Verification items for the finished model (mm, model axes). Face numbers are marked on the shaded views. A direction names the side the tool comes from. Coordinates: 2 decimals unless noted, no trailing zeros. Order: outer loops, then holes, each group sorted by start corner. A loop starts at its lowest first (then second) coordinate and runs counter-clockwise, first axis right, second up. Notation, with made-up numbers: M 54.25,49.25 L 73.25,49.25 A31 ccw 73.25,88.25 Z; hole C -29.5,-1.75 d4. An arc over 180 degrees is marked long. Return JSON: item names as keys, results as strings. Group by question number.
Q1. Access from +Z, -Z, +X, -X, +Y, -Y to the whole of each face (thin tool, end or side, straight path). Record for the marked faces 5, 6 and 7.
Q2. Section check C-C, the plane z = 2.25. Enter the section's corners in (x, y) (3 decimals).
Q3. Section check A-A, the plane y = -11. Enter the section's corners in (x, z), then the cut area to 3 significant figures.
Q4. Section check D-D, the plane x = 16. Enter the section's corners in (y, z) (3 decimals).
Q5. Thickness scan on probe 1 along Y at (x, z) = (-8, 15.25) (3 decimals); probe 2 along Y at (x, z) = (-12.5, 3.5) (3 decimals); probe 3 along Z at (x, y) = (8.5, 11). Record the ranges inside material, lowest first.
Q6. Mould release check, pull along X, two halves, no side actions. Record for the marked faces 1, 2, 3 and 4: pulls with the +X half, pulls with the -X half, needs draft (parallel to the pull), parting line crosses it, or undercut.
Q7. Go/stop test with flat-tipped pins: pin 1 Ø20 at (x, y) = (-9, -1.5) entering from +Z; pin 2 Ø8 at (y, z) = (-21.5, 9.5) entering from -X; pin 3 Ø0.7 at (x, z) = (-18.5, 0.5) entering from +Y; pin 4 Ø5.5 at (x, z) = (-12, 6.5) entering from -Y (3 decimals). Record where each tip stops, or that it passes through.
Q8. Section check B-B, the plane z = 9.75. Enter the section's corners in (x, y) (3 decimals).
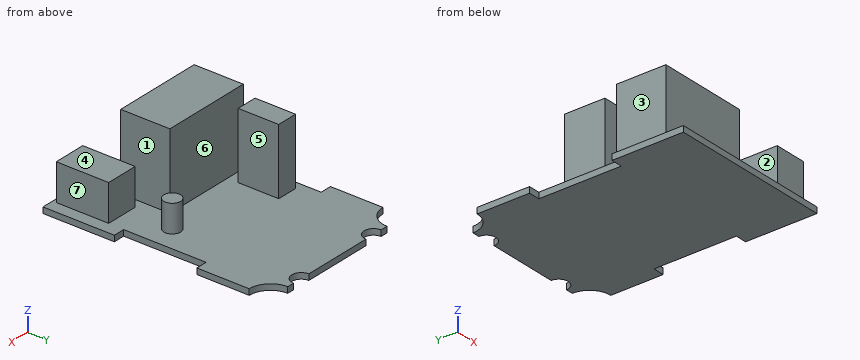
from build123d import *

# Parameters (mm, degrees)
F1_DEPTH = 1.44
F2_W     = 22.2
F2_H     = 12
F3_DEPTH = 18.42
F2_W_2   = 5.1
F2_H_2   = 9.9
F4_DEPTH = 16.2
F2_W_3   = 8
F2_H_3   = 12.8
F5_DEPTH = 8.9
F2_R     = 2.038774
F6_DEPTH = 6.7


with BuildPart() as f1:
    # F0 (on Top) → F1 (new body)
    with BuildSketch(Plane.XY):
        with BuildLine():
            Line((-20.21, -27.775), (20.21, -27.775))
            Line((20.21, -27.775), (20.21, -10.355))
            Line((20.21, -10.355), (17.41, -10.355))
            Line((17.41, -10.355), (17.41, 9.775))
            Line((17.41, 9.775), (20.21, 9.775))
            Line((20.21, 9.775), (20.21, 22.575))
            ThreePointArc((20.21, 22.575), (16.533045, 24.098045), (15.01, 27.775))
            Line((15.01, 27.775), (13.23, 27.775))
            ThreePointArc((13.23, 27.775), (10.93, 25.475), (8.63, 27.775))
            Line((8.63, 27.775), (-8.63, 27.775))
            ThreePointArc((-8.63, 27.775), (-10.93, 25.475), (-13.23, 27.775))
            Line((-13.23, 27.775), (-15.01, 27.775))
            ThreePointArc((-15.01, 27.775), (-16.533045, 24.098045), (-20.21, 22.575))
            Line((-20.21, 22.575), (-20.21, 9.775))
            Line((-20.21, 9.775), (-17.41, 9.775))
            Line((-17.41, 9.775), (-17.41, -10.355))
            Line((-17.41, -10.355), (-20.21, -10.355))
            Line((-20.21, -10.355), (-20.21, -27.775))
        make_face()
    extrude(amount=F1_DEPTH)

    # F2 (on face) → F3 (join)
    with BuildSketch(Plane.XY.offset(1.44)):
        with Locations((-4.11, -13.475)):
            Rectangle(F2_W, F2_H)
    extrude(amount=F3_DEPTH)

    # F2 (on face) → F4 (join)
    with BuildSketch(Plane.XY.offset(1.44)):
        with Locations((-12.93, 0.135)):
            Rectangle(F2_W_2, F2_H_2)
    extrude(amount=F4_DEPTH)

    # F2 (on face) → F5 (join)
    with BuildSketch(Plane.XY.offset(1.44)):
        with Locations((13.31, -20.475)):
            Rectangle(F2_W_3, F2_H_3)
    extrude(amount=F5_DEPTH)

    # F2 (on face) → F6 (join)
    with BuildSketch(Plane.XY.offset(1.44)):
        with Locations((11.359598, -3.366856)):
            Circle(F2_R)
    extrude(amount=F6_DEPTH)


solid = f1.part
Numbers:
{
 "1": {"face 5": "+Z, +Y", "face 6": "+Z, +X, -X", "face 7": "+Z, +X, +Y, -Y"},
 "2": {"outline": "M -15.48,-4.815 L -10.38,-4.815 L -10.38,5.085 L -15.48,5.085 Z; M -15.21,-19.475 L 6.99,-19.475 L 6.99,-7.475 L -15.21,-7.475 Z; M 9.31,-26.875 L 17.31,-26.875 L 17.31,-14.075 L 9.31,-14.075 Z; C 11.36,-3.367 d4.078"},
 "3": {"outline": "M -20.21,0 L 20.21,0 L 20.21,1.44 L 6.99,1.44 L 6.99,19.86 L -15.21,19.86 L -15.21,1.44 L -20.21,1.44 Z", "area": "467 mm2"},
 "4": {"outline": "M -27.775,0 L 24.723,0 L 24.723,1.44 L -14.075,1.44 L -14.075,10.34 L -26.875,10.34 L -26.875,1.44 L -27.775,1.44 Z"},
 "5": {"probe 1": "y = -19.475 to -7.475", "probe 2": "y = -19.475 to -7.475, -4.815 to 5.085", "probe 3": "z = 0 to 1.44"},
 "6": {"face 1": "undercut", "face 2": "undercut", "face 3": "pulls with the -X half", "face 4": "needs draft"},
 "7": {"pin 1": "stops at z = 19.86", "pin 2": "stops at x = -15.21", "pin 3": "stops at y = 23", "pin 4": "stops at y = -19.475"},
 "8": {"outline": "M -15.48,-4.815 L -10.38,-4.815 L -10.38,5.085 L -15.48,5.085 Z; M -15.21,-19.475 L 6.99,-19.475 L 6.99,-7.475 L -15.21,-7.475 Z; M 9.31,-26.875 L 17.31,-26.875 L 17.31,-14.075 L 9.31,-14.075 Z"}
}
